Input: part model. Units: mm. Frame: model coordinates. A direction names the side the tool comes from. Give positions to 0.01 mm unless a question says otherwise; leave off trailing zeros. Loops run counter-clockwise (first coordinate to the right, second up) from the corner with the lowest first, then second, coordinate; pieces in that order, holes last. Notation, with made-up numbers: M 87.5,83.25 L 118.5,83.25 A27 cw 118.5,99.25 Z; hole C -31,21.5 d7. An arc over 180 degrees is marked long. Use CSV: the item, a comma, the result in double quotes. Start each with the question number.
Q1. Pin query (flat end, axial travel): pin 1 (8 mm diameter, centred on x = 743.5, z = 129.5, fed in from +Y); pin 2 (23 mm diameter, centred on x = 1459, y = 175.5, fed in from -Z); pin 3 (5 mm diameter, centred on x = 1105, z = 52, fed in from +Y). Return the tip coordinate at first contact, or that it passes through.
Q2. Reachability of faces 4 (the flat face through (1151, -21.072, 97)), 5 (the flat face through (2056, 10, 8)), 6 (the flat face through (100, 2, 60)) from +Z, -Z, +X, -X, +Y, -Y: full face, straight path, thin tool, end or side. Return the list, or none.
Q3. Section A-A, the plane x = 915. Output: boundary loops of the cut face in (y, z), plus the area to 3 significant figures.
Q4. Pull-direction query (Z, two-part tool) for faces 1 (the flat face through (180, 10, 49.625)), 2 (the flat face through (1152, 48.928, 23)), 3 (the flat face through (1152, 14, 61.625)); classes: released by +Z, released by -Z, zero draft, split by the parting line, or undercut.
Q5. Material intervals for line 1 along Y through (x, z) = (1582, 134.5); line 2 along Z through (x, y) = (1778.5, -17); line 3 along Z through (x, y) = (847.5, 22.5), sorted ascending.
Q6. Section B-B, the plane y = 92.5. Output: boundary loops of the cut face in (x, z).
from build123d import *

# Parameters (mm, degrees)
F1_DEPTH = 2334
F2_W     = 278
F2_H     = 26
F3_DEPTH = 80
F4_DEPTH = 80


with BuildPart() as f1:
    # F0 (on Right) → F1 (new body)
    with BuildSketch(Plane.YZ):
        with BuildLine():
            Line((181.927831, 113.625399), (181.927831, 119.625399))
            Line((181.927831, 119.625399), (161.927831, 119.625399))
            ThreePointArc((161.927831, 119.625399), (158.392297, 121.089865), (156.927831, 124.625399))
            Line((156.927831, 124.625399), (156.927831, 134.625399))
            ThreePointArc((156.927831, 134.625399), (153.998899, 141.696467), (146.927831, 144.625399))
            Line((146.927831, 144.625399), (-17.072169, 144.625399))
            ThreePointArc((-17.072169, 144.625399), (-24.143237, 141.696467), (-27.072169, 134.625399))
            Line((-27.072169, 134.625399), (-27.072169, 61.625399))
            Line((-27.072169, 61.625399), (-21.072169, 61.625399))
            Line((-21.072169, 61.625399), (-21.072169, 133.625399))
            ThreePointArc((-21.072169, 133.625399), (-19.607703, 137.160933), (-16.072169, 138.625399))
            Line((-16.072169, 138.625399), (145.927831, 138.625399))
            ThreePointArc((145.927831, 138.625399), (149.463365, 137.160933), (150.927831, 133.625399))
            Line((150.927831, 133.625399), (150.927831, 123.625399))
            ThreePointArc((150.927831, 123.625399), (153.856763, 116.554331), (160.927831, 113.625399))
            Line((160.927831, 113.625399), (181.927831, 113.625399))
        make_face()
        with BuildLine():
            Line((-21.072169, 61.625399), (-27.072169, 61.625399))
            Line((-27.072169, 61.625399), (-27.072169, -4.374601))
            ThreePointArc((-27.072169, -4.374601), (-24.143237, -11.445669), (-17.072169, -14.374601))
            Line((-17.072169, -14.374601), (48.927831, -14.374601))
            Line((48.927831, -14.374601), (48.927831, -8.374601))
            Line((48.927831, -8.374601), (48.927831, 61.625399))
            Line((48.927831, 61.625399), (-21.072169, 61.625399))
        make_face()
    extrude(amount=F1_DEPTH)

    # F2 (on face) → F3 (cut)
    with BuildSketch(Plane.XZ.offset(27.072169)):
        with Locations((139, -17.374601)):
            Rectangle(F2_W, F2_H)
        with BuildLine():
            Line((95, 93.625399), (0, 93.625399))
            Line((0, 93.625399), (0, -4.374601))
            Line((0, -4.374601), (278, -4.374601))
            Line((278, -4.374601), (278, 29.625399))
            ThreePointArc((278, 29.625399), (272.142136, 43.767535), (258, 49.625399))
            Line((258, 49.625399), (100, 49.625399))
            Line((100, 49.625399), (100, 88.625399))
            ThreePointArc((100, 88.625399), (98.535534, 92.160933), (95, 93.625399))
        make_face()
    extrude(amount=-F3_DEPTH, mode=Mode.SUBTRACT)

    # F2 (on face) → F4 (cut)
    with BuildSketch(Plane.XZ.offset(27.072169)):
        with BuildLine():
            Line((2056, 29.625399), (2056, -4.374601))
            Line((2056, -4.374601), (2334, -4.374601))
            Line((2334, -4.374601), (2334, 93.625399))
            Line((2334, 93.625399), (2239, 93.625399))
            ThreePointArc((2239, 93.625399), (2235.464466, 92.160933), (2234, 88.625399))
            Line((2234, 88.625399), (2234, 49.625399))
            Line((2234, 49.625399), (2076, 49.625399))
            ThreePointArc((2076, 49.625399), (2061.857864, 43.767535), (2056, 29.625399))
        make_face()
        Polygon((2334, -4.374601), (2056, -4.374601), (2056, -14.374601), (2056, -32.294646), (2334, -32.294646), align=None)
    extrude(amount=-F4_DEPTH, mode=Mode.SUBTRACT)


solid = f1.part
A:
1,pin 1,"y = 156.93"
1,pin 2,"z = 113.63"
1,pin 3,"y = 48.93"
2,face 4,"+X, -X"
2,face 5,"-Z, +X, +Y, -Y"
2,face 6,"-Z, -X, +Y, -Y"
3,outline,"M -27.07,-4.37 A10 ccw -17.07,-14.37 L 48.93,-14.37 L 48.93,61.63 L -21.07,61.63 L -21.07,133.63 A5 cw -16.07,138.63 L 145.93,138.63 A5 cw 150.93,133.63 L 150.93,123.63 A10 ccw 160.93,113.63 L 181.93,113.63 L 181.93,119.63 L 161.93,119.63 A5 cw 156.93,124.63 L 156.93,134.63 A10 ccw 146.93,144.63 L -17.07,144.63 A10 ccw -27.07,134.63 Z"
3,area,"7,570 mm^2"
4,face 1,"released by -Z"
4,face 2,"zero draft"
4,face 3,"undercut"
5,line 1,"-27.07 to -21, 150.85 to 156.93"
5,line 2,"-14.37 to 61.63, 138.54 to 144.63"
5,line 3,"-14.37 to 61.63, 138.63 to 144.63"
6,outline,"M 0,138.63 L 2334,138.63 L 2334,144.63 L 0,144.63 Z"
